Autodesk Inventor part; units mm, degrees
ref_plane "YZ Plane" through (0, 0, 0) normal (1, 0, 0) x (0, 1, 0)
ref_plane "XZ Plane" through (0, 0, 0) normal (0, 1, 0) x (-1, 0, 0)
ref_plane "XY Plane" through (0, 0, 0) normal (0, 0, 1) x (1, 0, 0)
sketch "スケッチ1" plane through (0, 0, 0) normal (0, 0, 1) x (1, 0, 0)
  arc A0 (-1.5776, 2.5517) -> (-0.4828, -2.9609) centre (0, 0) ccw
  line L0 (-1.5776, 2.5517) -> (13.2904, 11.7436)
  line L1 (20.7039, 7.4628) -> (11.1913, -3.8738)
  line L2 (9.3374, -4.5621) -> (-0.4828, -2.9609)
  arc A1 (20.7039, 7.4628) -> (19.6894, 10.6802) centre (19.1718, 8.7484) ccw
  arc A2 (9.3374, -4.5621) -> (11.1913, -3.8738) centre (9.6593, -2.5882) ccw
  line L3 (0, 0) -> (9.6593, -2.5882)
  line L4 (9.6593, -2.5882) -> (19.1718, 8.7484)
  line L5 (-8.5052, 0) -> (26.6017, 0)
  line L6 (19.6894, 10.6802) -> (14.8598, 11.9743)
  arc A3 (14.8598, 11.9743) -> (13.2904, 11.7436) centre (14.3421, 10.0425) ccw
  line L7 (19.1718, 8.7484) -> (14.3421, 10.0425)
  line L8 (14.3421, 10.0425) -> (0, 0)
  dimension "d0" = 2
  dimension "d18" = 15
  dimension "d19" = 115
  dimension "d20" = 3
  dimension "d21" = 2
  dimension "d22" = 130
  dimension "d23" = 65
  dimension "d24" = 10
  dimension "d25" = 5
extrude "押し出し1" add sketch "スケッチ1" along normal blind 6.5
sketch "スケッチ3" plane through (0, 0, 6.5) normal (0, 0, 1) x (1, 0, 0)
  line L0 (0, 0) -> (1, 0) construction
  line L1 (0, 1.5) -> (1, 1.5)
  line L2 (1, -1.5) -> (0, -1.5)
  arc A0 (0, 1.5) -> (0, -1.5) centre (0, 0) ccw
  arc A1 (1, -1.5) -> (1, 1.5) centre (1, 0) ccw
  point P0 (0.5, 0)
  dimension "d7" = 3
  dimension "d8" = 1
extrude "押し出し3" cut sketch "スケッチ3" against normal through all
sketch "スケッチ5" plane through (0, 0, 6.5) normal (0, 0, 1) x (1, 0, 0)
  circle A0 centre (10, 0) radius 1.5
  line L0 (-7.8344, 0) -> (26.0061, 0)
  point P0 (0, 0)
  dimension "d14" = 3
  dimension "d15" = 10
extrude "押し出し5" cut sketch "スケッチ5" against normal through all
fillet "フィレット2" radius 1 16 edges at (-2.9425, -0.5844, 6.5) (4.4273, -3.7615, 6.5) (10.3554, -4.4631, 6.5) (15.9476, 1.7945, 6.5) (21.0792, 9.3498, 6.5) (17.2746, 11.3273, 6.5) (14.0513, 12.0212, 6.5) (5.8564, 7.1477, 6.5) (-2.9425, -0.5844, 0) (4.4273, -3.7615, 0) (10.3554, -4.4631, 0) (15.9476, 1.7945, 0) (21.0792, 9.3498, 0) (17.2746, 11.3273, 0) (14.0513, 12.0212, 0) (5.8564, 7.1477, 0)
properties part number "brake"
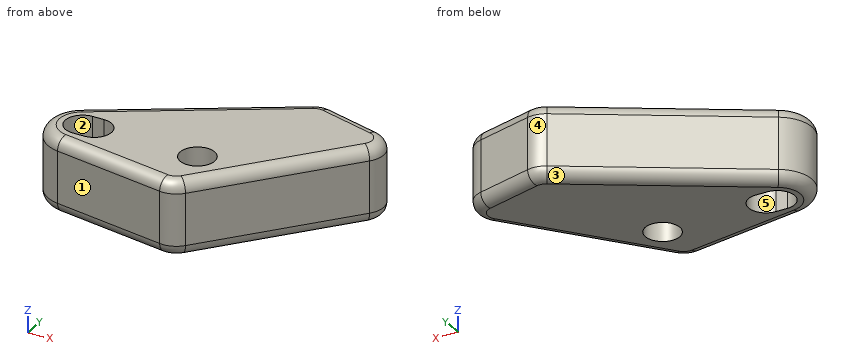
Can you work these out from the model? Positions are in its coordinate system, mm. Face numbers are marked on the shaded views. A direction names the side the tool comes from. Give positions to 0.01 mm unless a question says otherwise; leave off trailing zeros. Order: outer loops, then holes, each group sorted by start corner. A loop starts at its lowest first (then second) coordinate and runs counter-clockwise, first axis right, second up. Notation, with made-up numbers: M 29.5,28.25 L 70.5,28.25 A17 ccw 70.5,43.25 Z; hole C 31.25,-23.5 d3. An arc over 180 degrees is marked long. Use a Markdown table: item, result. Add a question column.
Item 1: Suppose I cut it at A-A (z = 1.5). List the corners of the cut face in (x, y) for me.
Item 2: For the marked faces 4 and 5, which set-ups out of +Z, -Z, +X, -X, +Y, -Y let a thin tool reach every point of the face, with its end or its side?
Item 3: We'd pull the mould along Y, two halves only. Please class the marked faces 1, 2 and 3: +Y half, -Y half, draft (parallel to the pull), parting line (faces both ways), or undercut.
Item 4: If I drill on L1, parallel to Y at x = 10, z = 5.25; L2, parallel to X at y = 0, z = 3.75; L3, parallel to X at y = -0.75, z = 4.5, over which ranges is the centre line in solid material (lowest first)? Write a range as [from, to].
Item 5: Will these pins go through, and if not, where does the flat tip stop? pin 1 (1 mm diameter, centred on x = 14, z = 0.5, fed in from +Y); pin 2 (0.8 mm diameter, centred on x = 0.5, z = 5, fed in from -Y); pin 3 (1.1 mm diameter, centred on x = 0.5, z = 2.5, fed in from +Y); pin 4 (2.5 mm diameter, centred on x = 10, y = 0, fed in from +Z).
Item 6: Suppose I cut it at B-B (y = 0). Count the separate pieces of the cut face and the enclosed holes in it, then the cut area to 3 significant figures.
Answer sheet:
| question | item | result |
|---|---|---|
| 1 | outline | M -1.58,2.55 A3 ccw -0.48,-2.96 L 9.34,-4.56 A2 ccw 11.19,-3.87 L 20.7,7.46 A2 ccw 19.69,10.68 L 14.86,11.97 A2 ccw 13.29,11.74 Z; hole M 0,-1.5 L 1,-1.5 A1.5 ccw 1,1.5 L 0,1.5 A1.5 ccw Z; hole C 10,0 d3 |
| 2 | face 4 | +Z, -Z, +Y |
| 2 | face 5 | +Z, -Z |
| 3 | face 1 | -Y half |
| 3 | face 2 | undercut |
| 3 | face 3 | +Y half |
| 4 | L1 | y = [-4.56, -1.5], [1.5, 9.71] |
| 4 | L2 | x = [-3, -1.5], [2.5, 8.5], [11.5, 14.44] |
| 4 | L3 | x = [-2.9, -1.3], [2.3, 8.7], [11.3, 13.81] |
| 5 | pin 1 | stops at y = 12.04 |
| 5 | pin 2 | stops at y = -3.19 |
| 5 | pin 3 | stops at y = 4.18 |
| 5 | pin 4 | passes through |
| 6 | separate pieces | 3 |
| 6 | enclosed holes | 0 |
| 6 | area | 66.9 mm² |
